from build123d import *

# Parameters (mm, degrees)
BOSS_EXTRUDE1_DEPTH  = 6
SKETCH4_R            = 20.1
CUT_EXTRUDE1_DEPTH   = 6
M5_CLEARANCE_HOLE1_D = 5.5
CUT_EXTRUDE2_DEPTH   = 6
M5_CLEARANCE_HOLE2_D = 5.5
CUT_EXTRUDE3_DEPTH   = 6


with BuildPart() as part:
    # Sketch3 → Boss-Extrude1 (new body)
    with BuildSketch(Plane.XY):
        with BuildLine():
            Line((-55, -75), (55, -75))
            ThreePointArc((55, -75), (58.535533906, -73.535533906), (60, -70))
            Line((60, -70), (60, 70))
            ThreePointArc((60, 70), (58.535533906, 73.535533906), (55, 75))
            Line((55, 75), (-55, 75))
            ThreePointArc((-55, 75), (-58.535533906, 73.535533906), (-60, 70))
            Line((-60, 70), (-60, -70))
            ThreePointArc((-60, -70), (-58.535533906, -73.535533906), (-55, -75))
        make_face()
    extrude(amount=BOSS_EXTRUDE1_DEPTH)

    # Sketch4 → Cut-Extrude1 (cut)
    with BuildSketch(Plane.XY.offset(6)):
        with Locations((0, -35)):
            Circle(SKETCH4_R)
    extrude(amount=-CUT_EXTRUDE1_DEPTH, mode=Mode.SUBTRACT)

    # M5 Clearance Hole1 (through all)
    with Locations(Plane.XY.offset(6)):
        with Locations((-23.57, -11.43), (23.57, -11.43), (23.57, -58.57), (-23.57, -58.57)):
            Hole(M5_CLEARANCE_HOLE1_D / 2)

    # Sketch7 → Cut-Extrude2 (cut)
    with BuildSketch(Plane.XY.offset(6)):
        with BuildLine():
            Line((-31.82, -11.43), (-31.82, -18.43))
            ThreePointArc((-31.82, -18.43), (-34.57, -21.18), (-37.32, -18.43))
            Line((-37.32, -18.43), (-37.32, -11.43))
            ThreePointArc((-37.32, -11.43), (-34.57, -8.68), (-31.82, -11.43))
        make_face()
        with BuildLine():
            Line((31.82, -11.43), (31.82, -18.43))
            ThreePointArc((31.82, -18.43), (34.57, -21.18), (37.32, -18.43))
            Line((37.32, -18.43), (37.32, -11.43))
            ThreePointArc((37.32, -11.43), (34.57, -8.68), (31.82, -11.43))
        make_face()
    extrude(amount=-CUT_EXTRUDE2_DEPTH, mode=Mode.SUBTRACT)

    # M5 Clearance Hole2 (through all)
    with Locations(Plane.XY.offset(6)):
        with Locations((-34.57, 46.47), (34.57, 46.47)):
            Hole(M5_CLEARANCE_HOLE2_D / 2)

    # Sketch10 → Cut-Extrude3 (cut)
    with BuildSketch(Plane.XY.offset(6)):
        with BuildLine():
            Line((-7.25, 63.5), (-7.25, 56.5))
            ThreePointArc((-7.25, 56.5), (-10, 53.75), (-12.75, 56.5))
            Line((-12.75, 56.5), (-12.75, 63.5))
            ThreePointArc((-12.75, 63.5), (-10, 66.25), (-7.25, 63.5))
        make_face()
        with BuildLine():
            Line((12.75, 63.5), (12.75, 56.5))
            ThreePointArc((12.75, 56.5), (10, 53.75), (7.25, 56.5))
            Line((7.25, 56.5), (7.25, 63.5))
            ThreePointArc((7.25, 63.5), (10, 66.25), (12.75, 63.5))
        make_face()
        with BuildLine():
            Line((-7.25, 29.44), (-7.25, 36.44))
            ThreePointArc((-7.25, 36.44), (-10, 39.19), (-12.75, 36.44))
            Line((-12.75, 36.44), (-12.75, 29.44))
            ThreePointArc((-12.75, 29.44), (-10, 26.69), (-7.25, 29.44))
        make_face()
        with BuildLine():
            Line((12.75, 29.44), (12.75, 36.44))
            ThreePointArc((12.75, 36.44), (10, 39.19), (7.25, 36.44))
            Line((7.25, 36.44), (7.25, 29.44))
            ThreePointArc((7.25, 29.44), (10, 26.69), (12.75, 29.44))
        make_face()
    extrude(amount=-CUT_EXTRUDE3_DEPTH, mode=Mode.SUBTRACT)


solid = part.part
Can you work these out from the model? Positions are in its coordinate system, mm. A direction names the side the tool comes from. Coordinates: 2 decimals unless noted, no trailing zeros. Order: outer loops, then holes, each group sorted by start corner. A loop starts at its lowest first (then second) coordinate and runs counter-clockwise, first axis right, second up. Notation, with made-up numbers: (-5, 45.25) - (18, 45.25) arc R23 ccw to (18, 84.25) - close; hole circle Ø2 at (57.25, -3.75). An arc over 180 degrees is marked (long way). Answer as a JSON object with one key per item and string values. Group by question number.
Q1. I need wall thicknesses on line 1 (X direction, y = 59, z = 2.1); line 2 (Y direction, x = 23.57, z = 4.65); line 3 (Y direction, x = -34.57, z = 3.1). Which ranges of each line are inside material? Lowest first, please. Write a range as from..to.
Q2. Imagine slicing it at B-B (y = -58.57). Please give me the cut outline in (x, z).
Q3. On a 3-axis mill with a long thin cutter (end or side, diameter ignored), from which of +Z, -Z, +X, -X, +Y, -Y can I reach the whole of each face in a straight line? I mean faces 5 (the face through (-34.51, -21.18, 3.04)), 6 (the face through (-1, 1, 0)). Say none if no direction works.
Q4. Will these pins go through, and if not, where does the flat tip stop? P1, Ø5, axis at x = -34.57, y = 46.47, coming from the -Z side; P2, Ø6.5, axis at x = 34.57, y = 46.47, coming from the +Z side.
Q5. Imagine slicing it at A-A (x = 0). Please give me the cut outline in (y, z), and give its area (3 significant figures).
Q6. Imagine slicing it at D-D (y = -16.5). Please give me the cut outline in (x, z).
Q7. We'd pull the mould along Y, two halves only. Please class faces 1 (the face through (58, -74, 3)), 2 (the face through (59, 73, 3)), 3 (the face through (-1, 1, 6)), 4 (the face through (12.75, 60, 3)): +Y half, -Y half, draft (parallel to the pull), parting line (faces both ways), or undercut.
Q8. Imagine slicing it at C-C (x = 34.57). Please give me the cut outline in (y, z), and give its area (3 significant figures).
Determined:
{
 "1": {"line 1": "x = -60..-12.75, -7.25..7.25, 12.75..60", "line 2": "y = -75..-61.32, -55.82..-14.18, -8.68..75", "line 3": "y = -75..-21.18, -8.68..43.72, 49.22..75"},
 "2": {"outline": "(-60, 0) - (-26.32, 0) - (-26.32, 6) - (-60, 6) - close; (-20.82, 0) - (20.82, 0) - (20.82, 6) - (-20.82, 6) - close; (26.32, 0) - (60, 0) - (60, 6) - (26.32, 6) - close"},
 "3": {"face 5": "+Z, -Z", "face 6": "-Z, +X, -X, +Y, -Y"},
 "4": {"P1": "passes through", "P2": "stops at z = 6"},
 "5": {"outline": "(-75, 0) - (-55.1, 0) - (-55.1, 6) - (-75, 6) - close; (-14.9, 0) - (75, 0) - (75, 6) - (-14.9, 6) - close", "area": "659 mm2"},
 "6": {"outline": "(-60, 0) - (-37.32, 0) - (-37.32, 6) - (-60, 6) - close; (-31.82, 0) - (-7.86, 0) - (-7.86, 6) - (-31.82, 6) - close; (7.86, 0) - (31.82, 0) - (31.82, 6) - (7.86, 6) - close; (37.32, 0) - (60, 0) - (60, 6) - (37.32, 6) - close"},
 "7": {"face 1": "-Y half", "face 2": "+Y half", "face 3": "draft", "face 4": "undercut"},
 "8": {"outline": "(-75, 0) - (-21.18, 0) - (-21.18, 6) - (-75, 6) - close; (-8.68, 0) - (43.72, 0) - (43.72, 6) - (-8.68, 6) - close; (49.22, 0) - (75, 0) - (75, 6) - (49.22, 6) - close", "area": "792 mm2"}
}
